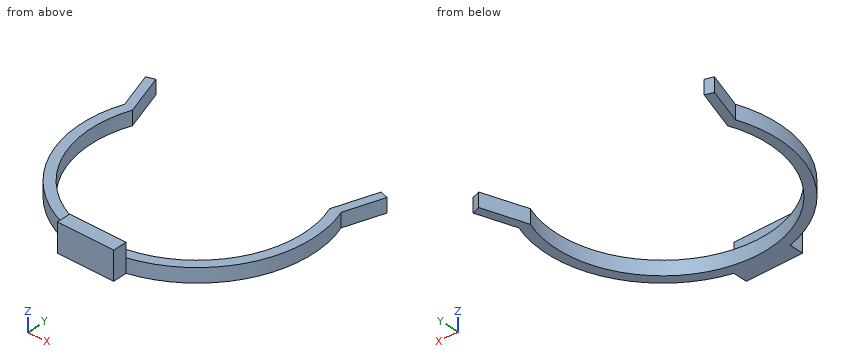
from build123d import *

# Parameters (mm, degrees)
PAD_DEPTH    = 5
SKETCH001_W  = 20
SKETCH001_H  = 5
PAD001_DEPTH = 5


with BuildPart() as part:
    # Sketch → Pad (new body)
    with BuildSketch(Plane.XY):
        with BuildLine():
            ThreePointArc((-35, 13.462912), (0, -37.5), (35, 13.462912))
            Line((35, 13.462912), (40, 28.462912))
            Line((40, 28.462912), (42.84605, 27.514229))
            Line((42.84605, 27.514229), (38.412275, 14.212903))
            ThreePointArc((10, -39.717873), (36.236297, -19.090317), (38.412275, 14.212903))
            Line((10, -44.717873), (10, -39.717873))
            Line((-10, -44.717873), (10, -44.717873))
            Line((-10, -39.717873), (-10, -44.717873))
            ThreePointArc((-38.412275, 14.212903), (-36.236297, -19.090317), (-10, -39.717873))
            Line((-42.84605, 27.514229), (-38.412275, 14.212903))
            Line((-42.84605, 27.514229), (-40, 28.462912))
            Line((-35, 13.462912), (-40, 28.462912))
        make_face()
    extrude(amount=PAD_DEPTH)

    # Sketch001 (on Face14 of Pad) → Pad001 (join)
    with BuildSketch(Plane.XY.offset(5)):
        with Locations((0, -42.217873)):
            Rectangle(SKETCH001_W, SKETCH001_H)
    extrude(amount=PAD001_DEPTH)


solid = part.part
Verification items for the finished model (mm, model axes). Give positions to 0.01 mm unless a question says otherwise; leave off trailing zeros. Loops run counter-clockwise (first coordinate to the right, second up) from the corner with the lowest first, then second, coordinate; pieces in that order, holes last. Notation, with made-up numbers: (85.25, -39.75) - (139.25, -39.75) arc R10 ccw to (139.25, -28.75) - close; hole circle Ø10 at (10.25, 50.5). An arc over 180 degrees is marked (long way). Write item = value, one per line. Start each with the question number.
Q1. Thickness scan on line 1 (X direction, y = 0, z = 1.35); line 2 (Y direction, x = 0, z = 2.7); line 3 (Z direction, x = 11.5, y = -36.5). Record the ranges inside material, lowest first.
Q2. Depth check by flat-ended pin: P1, Ø6, axis at y = -2.5, z = 6.5, coming from the +X side; P2, Ø1, axis at x = -1, z = 9, coming from the +Y side; P3, Ø2, axis at y = 10, z = 2.5, coming from the -X side. Enter the tip coordinate at first touch or a pass-through.
Q3. Cross-section at C-C, the plane x = 0. Enter the section's corners in (y, z), and give its area (3 significant figures).
Q4. Cross-section at A-A, the plane y = 0. Enter the section's corners in (x, z), and give its area (3 significant figures).
Q5. Cross-section at B-B, the plane z = 3. Enter the section's corners in (x, y).
Q6. Cross-section at D-D, the plane y = 20. Enter the section's corners in (x, z).
Answer key:
q1.line_1 = -40.96 to -37.5, 37.5 to 40.96
q1.line_2 = -44.72 to -37.5
q1.line_3 = 0 to 5
q2.P1 = 40.96
q2.P2 = -39.72
q2.P3 = -39.96
q3.outline = (-44.72, 0) - (-37.5, 0) - (-37.5, 5) - (-39.72, 5) - (-39.72, 10) - (-44.72, 10) - close
q3.area = 61.1 mm^2
q4.outline = (-40.96, 0) - (-37.5, 0) - (-37.5, 5) - (-40.96, 5) - close; (37.5, 0) - (40.96, 0) - (40.96, 5) - (37.5, 5) - close
q4.area = 34.6 mm^2
q5.outline = (-42.85, 27.51) - (-38.41, 14.21) arc R40.96 ccw to (-10, -39.72) - (-10, -44.72) - (10, -44.72) - (10, -39.72) arc R40.96 ccw to (38.41, 14.21) - (42.85, 27.51) - (40, 28.46) - (35, 13.46) arc R37.5 cw (long way) to (-35, 13.46) - (-40, 28.46) - close
q6.outline = (-40.34, 0) - (-37.18, 0) - (-37.18, 5) - (-40.34, 5) - close; (37.18, 0) - (40.34, 0) - (40.34, 5) - (37.18, 5) - close
